from build123d import *

# Parameters (mm, degrees)
SALIENTE_EXTRUIR1_DEPTH = 10
CROQUIS2_R              = 3.05
CORTAR_EXTRUIR1_DEPTH   = 34.103958495
SALIENTE_EXTRUIR2_START = 10
CROQUIS3_R              = 5.05
CROQUIS3_R_2            = 3.05
SALIENTE_EXTRUIR2_DEPTH = 10


with BuildPart() as part:
    # Croquis1 → Saliente-Extruir1 (new, symmetric)
    with BuildSketch(Plane(origin=(0, 0, 0), x_dir=(0, 0, -1), z_dir=(1, 0, 0))):
        with BuildLine():
            Line((-9.05, 0), (9.05, 0))
            Line((9.05, 0), (9.05, -23.257203825))
            Line((9.05, -23.257203825), (14.05, -23.257203825))
            Line((14.05, -23.257203825), (14.05, 3))
            ThreePointArc((14.05, 3), (13.464213562, 4.414213562), (12.05, 5))
            Line((12.05, 5), (-12.05, 5))
            ThreePointArc((-12.05, 5), (-13.464213562, 4.414213562), (-14.05, 3))
            Line((-14.05, 3), (-14.05, -23.257203825))
            Line((-14.05, -23.257203825), (-9.05, -23.257203825))
            Line((-9.05, -23.257203825), (-9.05, 0))
        make_face()
    extrude(amount=SALIENTE_EXTRUIR1_DEPTH, both=True)

    # Croquis2 → Cortar-Extruir1 (cut, through all)
    with BuildSketch(Plane(origin=(0, 5, 0), x_dir=(1, 0, 0), z_dir=(0, 1, 0))):
        with Locations(Location((0, 0, 0), (0, 0, 270))):
            Circle(CROQUIS2_R)
    extrude(amount=-CORTAR_EXTRUIR1_DEPTH, mode=Mode.SUBTRACT)

    # Croquis3 → Saliente-Extruir2 (add)
    with BuildSketch(Plane(origin=(0, 5, 0), x_dir=(1, 0, 0), z_dir=(0, 1, 0)).offset(SALIENTE_EXTRUIR2_START)):
        with Locations(Location((0, 0, 0), (0, 0, 90))):
            Circle(CROQUIS3_R)
        with Locations(Location((0, 0, 0), (0, 0, 270))):
            Circle(CROQUIS3_R_2, mode=Mode.SUBTRACT)
    extrude(amount=-SALIENTE_EXTRUIR2_DEPTH)


solid = part.part
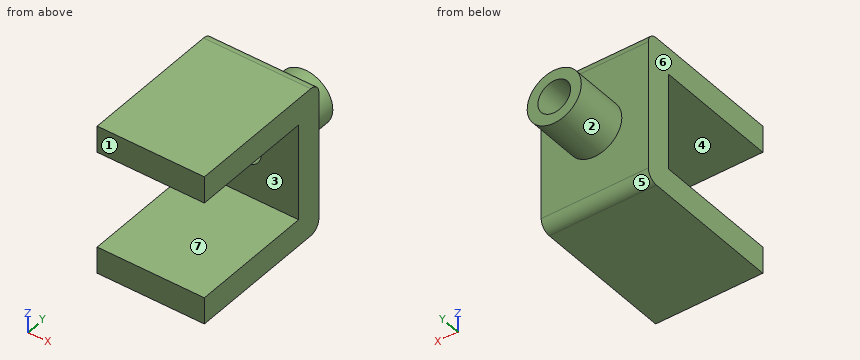
Could you check a few things on this model? Use its own coordinates, in mm. Face numbers are marked on the shaded views. A direction names the side the tool comes from. Round coordinates to 2 decimals unless told otherwise and drop trailing zeros. Write each loop counter-clockwise with the first axis right and the second up, starting at its lowest first coordinate (ties: lowest second). Pieces come first, ordered by that corner, then holes. Notation, with made-up numbers: (5.25, 74.5) - (18.25, 74.5) arc R15 cw to (18.25, 101.5) - close; hole circle Ø6 at (13.25, -3). An arc over 180 degrees is marked (long way). Put each result on its own line as item: value. Start each with the question number.
(1) Thinking about a two-plate mould opening in Z: for the marked faces 4, 5, 6 and 7, which applies, released by +Z, released by -Z, zero draft, split by the parting line, or undercut?
(2) I want a section at A-A, the plane z = 0. Please give me the cut outline in (x, y).
(3) I want a section at C-C, the plane y = -6.5. Please give me the cut outline in (x, z).
(4) I want a section at B-B, the plane x = 0. Please give me the cut outline in (y, z), plus the area to 3 significant figures.
(5) I need wall thicknesses on probe 1 along Z at (x, y) = (0, -17); probe 2 along X at (y, z) = (5.5, 0); probe 3 along X at (y, z) = (4.75, 0). Which ranges of each line are inside material? Lowest first, please.
(6) Will these pins go through, and if not, where does the flat tip stop? pin 1 (9 mm diameter, centred on x = -1.5, z = 3.5, fed in from -Y); pin 2 (2 mm diameter, centred on y = 9.5, z = -1, fed in from +X); pin 3 (6 mm diameter, centred on x = -8, z = 4.5, fed in from +Y); pin 4 (5 mm diameter, centred on x = 0, z = 0, fed in from -Y).
(7) I want a section at D-D, the plane x = 6.5. Please give me the cut outline in (y, z).
(8) For the marked faces 1, 2 and 3, which set-ups out of +Z, -Z, +X, -X, +Y, -Y let a thin tool reach every point of the face, with its end or its side?
Here are the results:
1. face 4: undercut
1. face 5: released by -Z
1. face 6: zero draft
1. face 7: undercut
2. outline: (-10, 0) - (-3.05, 0) - (-3.05, 15) - (-5.05, 15) - (-5.05, 5) - (-10, 5) - close; (3.05, 0) - (10, 0) - (10, 5) - (5.05, 5) - (5.05, 15) - (3.05, 15) - close
3. outline: (-10, -14.05) - (10, -14.05) - (10, -9.05) - (-10, -9.05) - close; (-10, 9.05) - (10, 9.05) - (10, 14.05) - (-10, 14.05) - close
4. outline: (-23.26, -14.05) - (3, -14.05) arc R2 ccw to (5, -12.05) - (5, -5.05) - (15, -5.05) - (15, -3.05) - (0, -3.05) - (0, -9.05) - (-23.26, -9.05) - close; (-23.26, 9.05) - (0, 9.05) - (0, 3.05) - (15, 3.05) - (15, 5.05) - (5, 5.05) - (5, 12.05) arc R2 ccw to (3, 14.05) - (-23.26, 14.05) - close
4. area: 381 mm^2
5. probe 1: z = -14.05 to -9.05, 9.05 to 14.05
5. probe 2: x = -5.05 to -3.05, 3.05 to 5.05
5. probe 3: x = -10 to -3.05, 3.05 to 10
6. pin 1: stops at y = 0
6. pin 2: stops at x = 5.05
6. pin 3: stops at y = 5
6. pin 4: passes through
7. outline: (-23.26, -14.05) - (3, -14.05) arc R2 ccw to (5, -12.05) - (5, 12.05) arc R2 ccw to (3, 14.05) - (-23.26, 14.05) - (-23.26, 9.05) - (0, 9.05) - (0, -9.05) - (-23.26, -9.05) - close
8. face 1: +Z, -Z, +X, -X, -Y
8. face 2: +Y
8. face 3: +X, -X, -Y
